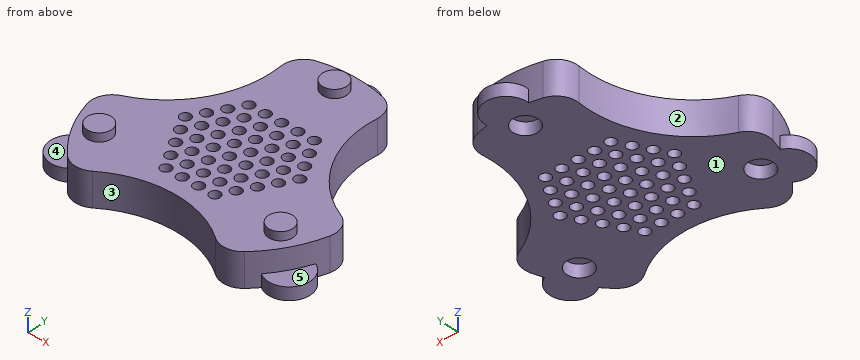
from build123d import *

# Parameters (mm, degrees)
SKETCH2_R           = 19
SKETCH2_R_2         = 1.25
SKETCH2_R_3         = 1.249999997
SKETCH2_R_4         = 1.250000002
SKETCH2_R_5         = 1.250000001
SKETCH2_R_6         = 1.249999999
SKETCH2_R_7         = 1.249999998
BOSS_EXTRUDE1_DEPTH = 8
SKETCH3_R           = 30
SKETCH3_R_2         = 17.487995661
BOSS_EXTRUDE2_DEPTH = 8
SKETCH4_R           = 2.9
BOSS_EXTRUDE3_DEPTH = 2
SKETCH6_R           = 5
BOSS_EXTRUDE4_DEPTH = 3
SKETCH5_R           = 3
CUT_EXTRUDE1_DEPTH  = 3
SKETCH7_R           = 25
CUT_EXTRUDE2_DEPTH  = 8
FILLET2_R           = 5


with BuildPart() as part:
    # Sketch2 → Boss-Extrude1 (new body)
    with BuildSketch(Plane.XY.offset(10)):
        Circle(SKETCH2_R)
        with Locations((0, -2.215732779)):
            Circle(SKETCH2_R_2, mode=Mode.SUBTRACT)
        with Locations((3.9, -2.215732779)):
            Circle(SKETCH2_R_2, mode=Mode.SUBTRACT)
        with Locations((7.8, -2.215732779)):
            Circle(SKETCH2_R_2, mode=Mode.SUBTRACT)
        with Locations((11.7, -2.215732779)):
            Circle(SKETCH2_R_2, mode=Mode.SUBTRACT)
        with Locations((1.95, -5.593231854)):
            Circle(SKETCH2_R_2, mode=Mode.SUBTRACT)
        with Locations((3.9, -8.970730929)):
            Circle(SKETCH2_R_2, mode=Mode.SUBTRACT)
        with Locations((5.850000003, -12.348230002)):
            Circle(SKETCH2_R_3, mode=Mode.SUBTRACT)
        with Locations((-1.95, -5.593231854)):
            Circle(SKETCH2_R_2, mode=Mode.SUBTRACT)
        with Locations((-3.9, -8.970730929)):
            Circle(SKETCH2_R_2, mode=Mode.SUBTRACT)
        with Locations((-5.85, -12.348230004)):
            Circle(SKETCH2_R_2, mode=Mode.SUBTRACT)
        with Locations((-3.9, -2.215732779)):
            Circle(SKETCH2_R_2, mode=Mode.SUBTRACT)
        with Locations((-7.8, -2.215732779)):
            Circle(SKETCH2_R_2, mode=Mode.SUBTRACT)
        with Locations((-11.7, -2.215732779)):
            Circle(SKETCH2_R_2, mode=Mode.SUBTRACT)
        with Locations((-1.950000001, 1.161766295)):
            Circle(SKETCH2_R_4, mode=Mode.SUBTRACT)
        with Locations((-3.9, 4.53926537)):
            Circle(SKETCH2_R_2, mode=Mode.SUBTRACT)
        with Locations((-5.85, 7.916764445)):
            Circle(SKETCH2_R_2, mode=Mode.SUBTRACT)
        with Locations((-7.8, 11.29426352)):
            Circle(SKETCH2_R_2, mode=Mode.SUBTRACT)
        with Locations((1.95, 1.161766295)):
            Circle(SKETCH2_R_5, mode=Mode.SUBTRACT)
        with Locations((3.9, 4.53926537)):
            Circle(SKETCH2_R_2, mode=Mode.SUBTRACT)
        with Locations((5.85, 7.916764445)):
            Circle(SKETCH2_R_2, mode=Mode.SUBTRACT)
        with Locations((7.8, 11.29426352)):
            Circle(SKETCH2_R_2, mode=Mode.SUBTRACT)
        with Locations((5.85, 1.161766295)):
            Circle(SKETCH2_R_2, mode=Mode.SUBTRACT)
        with Locations((7.8, 4.53926537)):
            Circle(SKETCH2_R_2, mode=Mode.SUBTRACT)
        with Locations((9.75, 1.161766295)):
            Circle(SKETCH2_R_2, mode=Mode.SUBTRACT)
        with Locations((11.7, 4.53926537)):
            Circle(SKETCH2_R_2, mode=Mode.SUBTRACT)
        with Locations((9.749099848, 7.918323553)):
            Circle(SKETCH2_R_2, mode=Mode.SUBTRACT)
        with Locations((13.650900152, 1.160207187)):
            Circle(SKETCH2_R_2, mode=Mode.SUBTRACT)
        with Locations((5.850000208, -5.594790783)):
            Circle(SKETCH2_R_2, mode=Mode.SUBTRACT)
        with Locations((9.750000208, -5.594790782)):
            Circle(SKETCH2_R_6, mode=Mode.SUBTRACT)
        with Locations((7.800000209, -8.972289857)):
            Circle(SKETCH2_R_7, mode=Mode.SUBTRACT)
        with Locations((-0.00134976, -8.973069502)):
            Circle(SKETCH2_R_2, mode=Mode.SUBTRACT)
        with Locations((1.94865024, -12.350568576)):
            Circle(SKETCH2_R_2, mode=Mode.SUBTRACT)
        with Locations((-1.95134976, -12.350568576)):
            Circle(SKETCH2_R_2, mode=Mode.SUBTRACT)
        with Locations((-5.852699936, -5.594791143)):
            Circle(SKETCH2_R_2, mode=Mode.SUBTRACT)
        with Locations((-7.802699936, -8.972290217)):
            Circle(SKETCH2_R_2, mode=Mode.SUBTRACT)
        with Locations((-9.752699936, -5.594791143)):
            Circle(SKETCH2_R_2, mode=Mode.SUBTRACT)
        with Locations((-5.852700144, 1.161765936)):
            Circle(SKETCH2_R_2, mode=Mode.SUBTRACT)
        with Locations((-9.752700144, 1.161765936)):
            Circle(SKETCH2_R_2, mode=Mode.SUBTRACT)
        with Locations((-7.802700144, 4.53926501)):
            Circle(SKETCH2_R_2, mode=Mode.SUBTRACT)
        with Locations((-11.702700144, 4.53926501)):
            Circle(SKETCH2_R_2, mode=Mode.SUBTRACT)
        with Locations((-9.751799992, 7.918323194)):
            Circle(SKETCH2_R_2, mode=Mode.SUBTRACT)
        with Locations((-13.653600295, 1.160206827)):
            Circle(SKETCH2_R_2, mode=Mode.SUBTRACT)
        with Locations((-0.001350176, 4.540044654)):
            Circle(SKETCH2_R_5, mode=Mode.SUBTRACT)
        with Locations((-1.951350176, 7.917543729)):
            Circle(SKETCH2_R_2, mode=Mode.SUBTRACT)
        with Locations((1.948649824, 7.917543729)):
            Circle(SKETCH2_R_2, mode=Mode.SUBTRACT)
        with Locations((-0.001350176, 11.295042804)):
            Circle(SKETCH2_R_2, mode=Mode.SUBTRACT)
        with Locations((3.900450128, 11.295042804)):
            Circle(SKETCH2_R_2, mode=Mode.SUBTRACT)
        with Locations((-3.903150479, 11.295042804)):
            Circle(SKETCH2_R_2, mode=Mode.SUBTRACT)
    extrude(amount=BOSS_EXTRUDE1_DEPTH)

    # Sketch3 → Boss-Extrude2 (add)
    with BuildSketch(Plane.XY.offset(18)):
        Circle(SKETCH3_R)
        Circle(SKETCH3_R_2, mode=Mode.SUBTRACT)
    extrude(amount=-BOSS_EXTRUDE2_DEPTH)

    # Sketch4 → Boss-Extrude3 (add)
    with BuildSketch(Plane.XY.offset(18)):
        with Locations((0, 25)):
            Circle(SKETCH4_R)
        with Locations((21.650635095, -12.5)):
            Circle(SKETCH4_R)
        with Locations((-21.650635095, -12.5)):
            Circle(SKETCH4_R)
    extrude(amount=BOSS_EXTRUDE3_DEPTH)

    # Sketch6 → Boss-Extrude4 (add)
    with BuildSketch(Plane(origin=(0, 0, 10), x_dir=(-1, 0, 0), z_dir=(0, 0, -1))):
        with Locations((0, 30)):
            Circle(SKETCH6_R)
        with Locations((25.980762114, -15)):
            Circle(SKETCH6_R)
        with Locations((-25.980762114, -15)):
            Circle(SKETCH6_R)
    extrude(amount=-BOSS_EXTRUDE4_DEPTH)

    # Sketch5 → Cut-Extrude1 (cut)
    with BuildSketch(Plane(origin=(0, 0, 10), x_dir=(-1, 0, 0), z_dir=(0, 0, -1))):
        with Locations((0, 25)):
            Circle(SKETCH5_R)
        with Locations((21.650635095, -12.5)):
            Circle(SKETCH5_R)
        with Locations((-21.650635095, -12.5)):
            Circle(SKETCH5_R)
    extrude(amount=-CUT_EXTRUDE1_DEPTH, mode=Mode.SUBTRACT)

    # Sketch7 → Cut-Extrude2 (cut)
    with BuildSketch(Plane(origin=(0, 0, 10), x_dir=(-1, 0, 0), z_dir=(0, 0, -1))):
        with Locations((36.373066959, 21)):
            Circle(SKETCH7_R)
        with Locations((0, -42)):
            Circle(SKETCH7_R)
        with Locations((-36.373066959, 21)):
            Circle(SKETCH7_R)
    extrude(amount=-CUT_EXTRUDE2_DEPTH, mode=Mode.SUBTRACT)

    # Fillet2
    fillet2_edges = [part.edges().sort_by_distance(p)[0] for p in [
        (29.836243213, -3.130270104, 14),
        (12.207228175, 27.404079628, 14),
        (-12.207228175, 27.404079628, 14),
        (-29.836243213, -3.130270104, 14),
        (-17.629015038, -24.273809524, 14),
        (17.629015038, -24.273809524, 14),
    ]]
    fillet(fillet2_edges, radius=FILLET2_R)


solid = part.part
The listing builds one solid part. Answer for the finished solid, in the listing's coordinates (mm). Face numbers are marked on the shaded views. A direction names the side the tool comes from. Give positions to 0.01 mm unless a question says otherwise; leave off trailing zeros. Loops run counter-clockwise (first coordinate to the right, second up) from the corner with the lowest first, then second, coordinate; pieces in that order, holes last. Notation, with made-up numbers: (86, 66) - (133, 66) arc R13 ccw to (133, 75) - close; hole circle Ø7 at (73.5, 86.25). An arc over 180 degrees is marked (long way). Use one line per item in the form item = value.
1. Which of the six approach directions +Z, -Z, +X, -X, +Y, -Y give full straight-line access (tool end or side, diameter ignored) to the marked faces 1, 2, 3, 4 and 5?
Calculated:
face_1 = -Z, +X, -X, +Y, -Y
face_2 = +Z, -Z, -X
face_3 = +Z, -Z, -Y
face_4 = +Z, -X, -Y
face_5 = +Z, +X, -Y
2. Section D-D on y = 20.5 is taken. Give the vertices of the cut face in (x, z), then the cut area to 3 significant figures.
Calculated:
outline = (-11.38, 10) - (11.38, 10) - (11.38, 18) - (-11.38, 18) - close
area = 182 mm^2
3. Section A-A on x = 0 is taken. Count the separate pieces of the cut face and the enclosed holes in it, then the cut area to 3 significant figures.
Calculated:
separate_pieces = 5
enclosed_holes = 0
area = 305 mm^2
4. Section B-B on x = -22 is taken. Give the vertices of the cut face in (y, z).
Calculated:
outline = (-20.4, 10) - (-15.48, 10) - (-15.48, 13) - (-9.52, 13) - (-9.52, 10) - (0.54, 10) - (0.54, 18) - (-9.62, 18) - (-9.62, 20) - (-15.38, 20) - (-15.38, 18) - (-20.4, 18) - close
5. Find the intervals of material crossed by line 1 along Y through (x, z) = (-6, 11); line 2 along Y through (x, z) = (-3.9, 15.75); line 3 along X through (y, z) = (-13, 16.75), in increasing order. Write a range as [from, to].
Calculated:
line_1 = [-17.73, -13.59], [-11.11, -6.84], [-4.35, -0.08], [2.4, 6.68], [9.16, 29.39]
line_2 = [-17.31, -10.22], [-7.72, -3.47], [-0.97, 3.29], [5.79, 10.05], [12.55, 29.75]
line_3 = [-27.04, -6.92], [-4.78, -3.02], [-0.88, 0.88], [3.02, 4.78], [6.92, 27.04]
6. Given pin 1 Ø2 at (x, y) = (11.7, -2.22) entering from -Z; pin 2 Ø1.5 at (y, z) = (3.5, 16.5) entering from +X; pin 3 Ø12 at (x, y) = (-11.5, -2.5) entering from +Z, each flat-ended and moving along its own axis, determine where each tip first touches the part or whether it passes through.
Calculated:
pin_1 = through
pin_2 = 19.29
pin_3 = 18
